Part model, mm, in its own coordinate system. Face numbers are marked on the shaded views. Round coordinates to 2 decimals unless told otherwise and drop trailing zeros. Write each loop counter-clockwise with the first axis right and the second up, starting at its lowest first coordinate (ties: lowest second). Pieces come first, ordered by that corner, then holes. Notation, with made-up numbers: (82, 54.5) -> (128, 54.5) arc R30 ccw to (128, 81.5) -> close; hole circle Ø11 at (-35.5, 41). An arc over 180 degrees is marked (long way). Return JSON: item names as keys, results as strings. Group by question number.
(1) Saw through at D-D (z = 1.75). List the corners of the cut face in (x, y) (3 decimals), plus the area to 3 significant figures.
(2) Drill centre lines: L1, parallel to Y at x = 4.5, z = 1 (3 decimals); L2, parallel to X at y = -1.5, z = 6.25; L3, parallel to X at y = 0.5, z = 1.75. Where is each one in solid material? Low to high. Write a range as from..to.
(3) Drop flat-ended pins along their axis: pin 1 Ø1.5 at (y, z) = (0.5, 3.5) entering from -X; pin 2 Ø0.7 at (x, y) = (4.5, 1) entering from +Z (3 decimals); pin 3 Ø1 at (x, y) = (6, -1) entering from +Z. Give the stop position or say it passes through.
(4) Mould opens along Y. For the marked faces 1, 2 and 3 say: +Y half, -Y half, draft (parallel to the pull), parting line (faces both ways), or undercut.
(5) Saw through at B-B (z = 3.5). List the corners of the cut face in (x, y) (3 decimals), plus the area to 3 significant figures.
(6) Saw through at C-C (x = 4.5). State how many separate pieces and enclosed holes the cut face has, plus the area to 3 significant figures.
(7) Saw through at A-A (y = -3.5). List the corners of the cut face in (x, z) (3 decimals), plus the area to 3 significant figures.
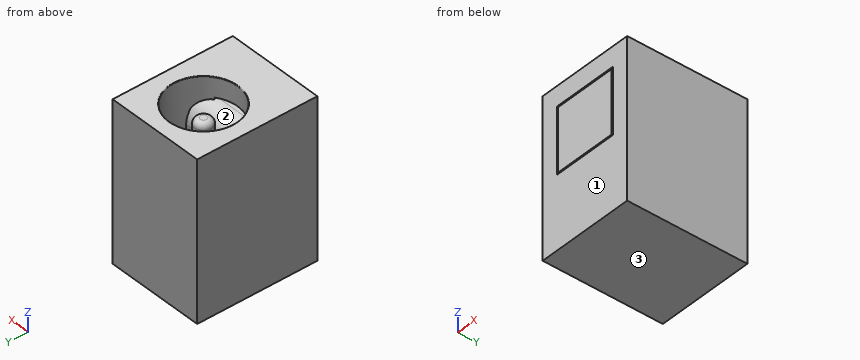
from build123d import *

# Parameters (mm, degrees)
ESBO_O1_W                     = 14.45
ESBO_O1_H                     = 11
RESSALTO_EXTRUS_O1_DEPTH      = 9
ESBO_O3_R                     = 3.125
CORTE_EXTRUS_O2_DEPTH         = 8.93
ESBO_O4_R                     = 0.8
RESSALTO_EXTRUS_O2_DEPTH      = 7.71
FILETE1_R                     = 0.5
FILETE2_R                     = 0.05
ESBO_O5_W                     = 6
ESBO_O5_H                     = 6
CORTE_EXTRUS_O5_DEPTH         = 4
RESSALTO_EXTRUS_O4_DEPTH      = 4
RESSALTO_EXTRUS_O4_DEPTH_BACK = 1.7
ESBO_O7_W                     = 5.688524138
ESBO_O7_H                     = 5.729720352
FILETE5_R                     = 2
CHANFRO4_SIZE                 = 2


with BuildPart() as part:
    # Esboço1 → Ressalto-extrusão1 (new body)
    with BuildSketch(Plane(origin=(0, 0, 0), x_dir=(0, 0, -1), z_dir=(1, 0, 0))):
        Rectangle(ESBO_O1_W, ESBO_O1_H)
    extrude(amount=RESSALTO_EXTRUS_O1_DEPTH)

    # Esboço3 → Corte-extrusão2 (cut)
    with BuildSketch(Plane.XY.offset(7.225)):
        with Locations((4.5, 1.05)):
            Circle(ESBO_O3_R)
    extrude(amount=-CORTE_EXTRUS_O2_DEPTH, mode=Mode.SUBTRACT)

    # Esboço4 → Ressalto-extrusão2 (add)
    with BuildSketch(Plane.XY.offset(-1.705)):
        with Locations(Location((4.5, 1.05, 0), (0, 0, 180))):
            Circle(ESBO_O4_R)
    extrude(amount=RESSALTO_EXTRUS_O2_DEPTH)

    # Filete1
    filete1_edges = [part.edges().sort_by_distance(p)[0] for p in [
        (5.3, 1.05, 6.005),
    ]]
    fillet(filete1_edges, radius=FILETE1_R)

    # Filete2
    filete2_edges = [part.edges().sort_by_distance(p)[0] for p in [
        (1.375, 1.05, 7.225),
    ]]
    fillet(filete2_edges, radius=FILETE2_R)

    # Esboço5 → Corte-extrusão5 (cut)
    with BuildSketch(Plane.XZ.offset(5.5)):
        with Locations((4.5, 2.425)):
            Rectangle(ESBO_O5_W, ESBO_O5_H)
    extrude(amount=-CORTE_EXTRUS_O5_DEPTH, mode=Mode.SUBTRACT)

    # Esboço7 → Ressalto-extrusão4 (add, two sides: drawn at the far end of the back side and taken through both)
    with BuildSketch(Plane.XZ.offset(1.5).offset(-RESSALTO_EXTRUS_O4_DEPTH_BACK)):
        with Locations((4.5, 2.425)):
            Rectangle(ESBO_O7_W, ESBO_O7_H)
    extrude(amount=RESSALTO_EXTRUS_O4_DEPTH + RESSALTO_EXTRUS_O4_DEPTH_BACK)

    # Filete5
    # the kernel refuses this fillet: 2 mm, written as the material it takes off along each edge
    with BuildSketch(Plane(origin=(12.344262069, 0.2, 5.289860176), x_dir=(0, -1, 0), z_dir=(-1, 0, 0))) as filete5_piece_1_section:
        with BuildLine():
            CenterArc((FILETE5_R, -FILETE5_R), FILETE5_R, 90, 90)
            Line((0, -FILETE5_R), (0, 0))
            Line((0, 0), (FILETE5_R, 0))
        make_face()
    filete5_piece_1 = extrude(amount=15.688524139, mode=Mode.PRIVATE)
    filete5_piece_1 = split(filete5_piece_1, bisect_by=Plane(origin=(6.764399642, -1.5, 5.283313475), z_dir=(0, -1, 0)), keep=Keep.TOP, mode=Mode.PRIVATE)
    filete5_piece_1 = split(filete5_piece_1, bisect_by=Plane(origin=(1.5, -1.579624939, 5.283313475), z_dir=(1, 0, 0)), keep=Keep.TOP, mode=Mode.PRIVATE)
    filete5_piece_1 = split(filete5_piece_1, bisect_by=Plane(origin=(7.5, -1.579624939, 5.283313475), z_dir=(-1, 0, 0)), keep=Keep.TOP, mode=Mode.PRIVATE)
    add(filete5_piece_1, mode=Mode.SUBTRACT)
    with BuildSketch(Plane(origin=(12.344262069, 0.2, 5.289860176), x_dir=(0, -1, 0), z_dir=(-1, 0, 0))) as filete5_piece_2_section:
        with BuildLine():
            CenterArc((FILETE5_R, -FILETE5_R), FILETE5_R, 90, 90)
            Line((0, -FILETE5_R), (0, 0))
            Line((0, 0), (FILETE5_R, 0))
        make_face()
    filete5_piece_2 = extrude(amount=15.688524139, mode=Mode.PRIVATE)
    filete5_piece_2 = filete5_piece_2 & Plane(origin=(4.5, 1.05, 4.831537274), x_dir=(1, 0, 0), z_dir=(0, 0, 1)) * Cylinder(3.125, 40, mode=Mode.PRIVATE)
    add(filete5_piece_2, mode=Mode.SUBTRACT)

    # Chanfro4
    # the kernel refuses this chamfer: 2 mm, written as the material it takes off along each edge
    with BuildSketch(Plane(origin=(-3.487628045, 0.2, -0.439860176), x_dir=(0, 0.02749587661058638, 0.9996219169112968), z_dir=(1, 0, 0))) as chanfro4_piece_1_section:
        Polygon((CHANFRO4_SIZE * 0.999621916911, CHANFRO4_SIZE * 0.0274958766106), (-CHANFRO4_SIZE * 0.0274958766106, CHANFRO4_SIZE * 0.999621916911), (0, 0), align=None)
    chanfro4_piece_1 = extrude(amount=15.975256091, mode=Mode.PRIVATE)
    chanfro4_piece_1 = split(chanfro4_piece_1, bisect_by=Plane(origin=(2.25835967, -1.5, -0.343331673), z_dir=(0, -1, 0)), keep=Keep.TOP, mode=Mode.PRIVATE)
    chanfro4_piece_1 = split(chanfro4_piece_1, bisect_by=Plane(origin=(7.5, -1.606942994, -0.343331673), z_dir=(-1, 0, 0)), keep=Keep.TOP, mode=Mode.PRIVATE)
    chanfro4_piece_1 = split(chanfro4_piece_1, bisect_by=Plane(origin=(1.5, -1.606942994, -0.343331673), z_dir=(1, 0, 0)), keep=Keep.TOP, mode=Mode.PRIVATE)
    add(chanfro4_piece_1, mode=Mode.SUBTRACT)
    with BuildSketch(Plane(origin=(-3.487628045, 0.2, -0.439860176), x_dir=(0, 0.02749587661058638, 0.9996219169112968), z_dir=(1, 0, 0))) as chanfro4_piece_2_section:
        Polygon((CHANFRO4_SIZE * 0.999621916911, CHANFRO4_SIZE * 0.0274958766106), (-CHANFRO4_SIZE * 0.0274958766106, CHANFRO4_SIZE * 0.999621916911), (0, 0), align=None)
    chanfro4_piece_2 = extrude(amount=15.975256091, mode=Mode.PRIVATE)
    chanfro4_piece_2 = chanfro4_piece_2 & Plane(origin=(4.5, 1.05, 0.259438948), x_dir=(1, 0, 0), z_dir=(0, 0, 1)) * Cylinder(3.125, 40, mode=Mode.PRIVATE)
    add(chanfro4_piece_2, mode=Mode.SUBTRACT)


solid = part.part
Computed values:
{
 "1": {"outline": "(0, -5.5) -> (1.5, -5.5) -> (1.5, -1.5) -> (1.656, -1.5) -> (1.656, -5.5) -> (7.344, -5.5) -> (7.344, -1.5) -> (7.5, -1.5) -> (7.5, -5.5) -> (9, -5.5) -> (9, 5.5) -> (0, 5.5) -> close; circle Ø1.6 at (4.5, 1.05); hole (1.656, -0.245) -> (1.656, 0.2) -> (7.344, 0.2) -> (7.344, -0.245) arc R3.125 ccw (long way) to start", "area": "79.1 mm2"},
 "2": {"L1": "-5.5..-0.36, 0.25..1.85, 4.175..5.5", "L2": "0..2.69, 6.31..9", "L3": "0..1.42, 3.92..5.08, 7.58..9"},
 "3": {"pin 1": "x = 0", "pin 2": "z = 6.005", "pin 3": "z = 5.27"},
 "4": {"face 1": "-Y half", "face 2": "undercut", "face 3": "draft"},
 "5": {"outline": "(0, -5.5) -> (1.5, -5.5) -> (1.5, -1.5) -> (1.656, -1.5) -> (1.656, -5.5) -> (7.344, -5.5) -> (7.344, -1.5) -> (7.5, -1.5) -> (7.5, -5.5) -> (9, -5.5) -> (9, 5.5) -> (0, 5.5) -> close; circle Ø1.6 at (4.5, 1.05); hole (1.656, -0.245) -> (1.656, 0.189) -> (7.344, 0.189) -> (7.344, -0.245) arc R3.125 ccw (long way) to start", "area": "79.0 mm2"},
 "6": {"separate pieces": "3", "enclosed holes": "0", "area": "125 mm2"},
 "7": {"outline": "(0, -7.225) -> (9, -7.225) -> (9, 7.225) -> (0, 7.225) -> close; (1.656, -0.44) -> (7.344, -0.44) -> (7.344, 5.29) -> (1.656, 5.29) -> close; hole (1.5, -0.575) -> (7.5, -0.575) -> (7.5, 5.425) -> (1.5, 5.425) -> close", "area": "127 mm2"}
}
